Design review of the part built by this model. Coordinates are the model's own, in mm. Face numbers are marked on the shaded views. Round coordinates to 2 decimals unless told otherwise and drop trailing zeros. Loops run counter-clockwise (first coordinate to the right, second up) from the corner with the lowest first, then second, coordinate; pieces in that order, holes last. Notation, with made-up numbers: M -24,20.5 L -6,20.5 A26 ccw -6,38.5 Z; hole C 18,51 d3. An arc over 180 degrees is marked long. One line per item, written item: value. Start each with the question number.
Item 1: We need section C-C (z = 7.5). Write out the cut boundary in (x, y).
Item 2: We need section D-D (x = 14). Write out the cut boundary in (y, z).
Item 3: Clearance check with flat-ended pins moving along their axes: pin 1 (6.5 mm diameter, centred on x = -16.5, y = 15.5, fed in from +Z); pin 2 (1 mm diameter, centred on x = 18.5, z = 12.5, fed in from +Y); pin 3 (3.5 mm diameter, centred on x = 0.5, z = 1.5, fed in from -Y); pin 4 (1.5 mm diameter, centred on y = -15, z = 11.5, fed in from -X). State where each tip first meets the part, or that it passes through.
Item 4: For line 1 along X through (y, z) = (-20.5, 13); line 2 along X through (y, z) = (21.5, 7.75); line 3 along Y through (x, z) = (24, 14), list the stretches that pass through material, from the lowest coordinate up.
Item 5: We need section B-B (z = 13.75). Write out the cut boundary in (x, y), then the cut area to 3 significant figures.
Item 6: Mouldability with a two-part tool opening along X and no side actions: class the marked faces 1 and 2 as released by +X, released by -X, zero draft, split by the parting line, or undercut.
Item 7: We need section A-A (y = 0). Write out the cut boundary in (x, z), then the cut area to 3 significant figures.
from build123d import *

# Parameters (mm, degrees)
F0_W      = 55
F0_H      = 55
F1_DEPTH  = 3
F2_R      = 3.5
F3_DEPTH  = 3
F4_R      = 2.9
F5_DEPTH  = 3
F6_R      = 4.5
F7_DEPTH  = 12
F8_R      = 3.2
F9_DEPTH  = 12
F10_R     = 4
F11_W     = 15
F11_H     = 15
F12_DEPTH = 20
F14_DEPTH = 25
F15_R     = 8
F16_R     = 5


with BuildPart() as f1:
    # F0 (on Top) → F1 (new body)
    with BuildSketch(Plane.XY):
        Rectangle(F0_W, F0_H)
    extrude(amount=F1_DEPTH)

    # F2 (on face) → F3 (join)
    with BuildSketch(Plane.XY.offset(3)):
        with Locations((-15.9099025767, 15.9099025767)):
            Circle(F2_R)
        with Locations((15.9099025767, 15.9099025767)):
            Circle(F2_R)
        with Locations((-15.9099025767, -15.9099025767)):
            Circle(F2_R)
        with Locations((15.9099025767, -15.9099025767)):
            Circle(F2_R)
    extrude(amount=F3_DEPTH)

    # F4 (on face) → F5 (join)
    with BuildSketch(Plane.XY.offset(6)):
        with Locations((-15.9099025767, 15.9099025767)):
            Circle(F4_R)
        with Locations((15.9099025767, 15.9099025767)):
            Circle(F4_R)
        with Locations((-15.9099025767, -15.9099025767)):
            Circle(F4_R)
        with Locations((15.9099025767, -15.9099025767)):
            Circle(F4_R)
    extrude(amount=F5_DEPTH)

    # F6 (on face) → F7 (join)
    with BuildSketch(Plane.XY.offset(3)):
        with Locations((-22.627416998, 22.627416998)):
            Circle(F6_R)
        with Locations((22.627416998, 22.627416998)):
            Circle(F6_R)
        with Locations((22.627416998, -22.627416998)):
            Circle(F6_R)
        with Locations((-22.627416998, -22.627416998)):
            Circle(F6_R)
    extrude(amount=F7_DEPTH)

    # F8 (on face) → F9 (cut)
    with BuildSketch(Plane.XY.offset(15)):
        with Locations((-22.627416998, -22.627416998)):
            Circle(F8_R)
        with Locations((22.627416998, -22.627416998)):
            Circle(F8_R)
        with Locations((-22.627416998, 22.627416998)):
            Circle(F8_R)
        with Locations((22.627416998, 22.627416998)):
            Circle(F8_R)
    extrude(amount=-F9_DEPTH, mode=Mode.SUBTRACT)

    # F10
    f10_edges = [f1.edges().sort_by_distance(p)[0] for p in [
        (27.5, -27.5, 1.5),
        (-27.5, -27.5, 1.5),
        (-27.5, 27.5, 1.5),
        (27.5, 27.5, 1.5),
    ]]
    fillet(f10_edges, radius=F10_R)

    # F11 (on face) → F12 (cut, symmetric)
    with BuildSketch(Plane.XY.offset(3)):
        Polygon((-12.5, 4.5), (-27.5, 19.5), (-27.5, -19.5), (-12.5, -4.5), align=None)
        Polygon((19.5, 27.5), (-19.5, 27.5), (-4.5, 12.5), (4.5, 12.5), align=None)
        Polygon((27.5, -19.5), (27.5, 19.5), (12.5, 4.5), (12.5, -4.5), align=None)
        Polygon((-4.5, -12.5), (-19.5, -27.5), (19.5, -27.5), (4.5, -12.5), align=None)
        Rectangle(F11_W, F11_H)
    extrude(amount=F12_DEPTH, both=True, mode=Mode.SUBTRACT)

    # F13 (on face) → F14 (cut)
    with BuildSketch(Plane.XY.offset(3)):
        Polygon((-26.8456843913, 19.823363167), (-25.4314708289, 18.4091496047), (-22.6030437041, 21.2375767294), (-24.0172572665, 22.6517902918), align=None)
        Polygon((22.6030437041, 21.2375767294), (25.4314708289, 18.4091496047), (26.8456843913, 19.823363167), (24.0172572665, 22.6517902918), align=None)
        Polygon((-25.4314708289, -18.4091496047), (-26.8456843913, -19.823363167), (-24.0172572665, -22.6517902918), (-22.6030437041, -21.2375767294), align=None)
        Polygon((26.8456843913, -19.823363167), (25.4314708289, -18.4091496047), (22.6030437041, -21.2375767294), (24.0172572665, -22.6517902918), align=None)
    extrude(amount=F14_DEPTH, mode=Mode.SUBTRACT)

    # F15
    f15_edges = [f1.edges().sort_by_distance(p)[0] for p in [
        (19.5, -27.5, 1.5),
        (4.5, -12.5, 1.5),
        (-4.5, -12.5, 1.5),
        (-19.5, -27.5, 1.5),
        (-27.5, -19.5, 1.5),
        (-12.5, -4.5, 1.5),
        (-12.5, 4.5, 1.5),
        (-27.5, 19.5, 1.5),
        (-19.5, 27.5, 1.5),
        (-4.5, 12.5, 1.5),
        (4.5, 12.5, 1.5),
        (19.5, 27.5, 1.5),
        (12.5, -4.5, 1.5),
        (12.5, 4.5, 1.5),
        (27.5, 19.5, 1.5),
        (27.5, -19.5, 1.5),
    ]]
    fillet(f15_edges, radius=F15_R)

    # F16
    f16_edges = [f1.edges().sort_by_distance(p)[0] for p in [
        (-7.5, 7.5, 1.5),
        (7.5, 7.5, 1.5),
        (7.5, -7.5, 1.5),
        (-7.5, -7.5, 1.5),
    ]]
    fillet(f16_edges, radius=F16_R)


solid = f1.part
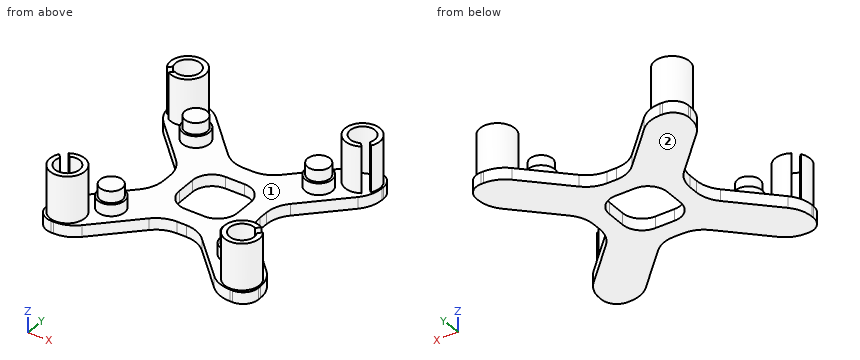
A:
1. outline: M -26.44,-20.23 A4.5 ccw long -25.02,-18.82 L -24.07,-19.77 A3.2 cw long -25.48,-21.19 Z; M -26.44,20.23 L -25.48,21.19 A3.2 cw long -24.07,19.77 L -25.02,18.82 A4.5 ccw long Z; C -15.91,-15.91 d5.8; C -15.91,15.91 d5.8; C 15.91,-15.91 d5.8; C 15.91,15.91 d5.8; M 24.07,-19.77 L 25.02,-18.82 A4.5 ccw long 26.44,-20.23 L 25.48,-21.19 A3.2 cw long Z; M 24.07,19.77 A3.2 cw long 25.48,21.19 L 26.44,20.23 A4.5 ccw long 25.02,18.82 Z
2. outline: M -22,0 L -5.85,0 L -5.85,3 L -12.98,3 L -12.98,6 L -13.73,6 L -13.73,9 L -18.09,9 L -18.09,6 L -18.84,6 L -18.84,3 L -22,3 Z; M 5.85,0 L 22,0 L 22,3 L 18.84,3 L 18.84,6 L 18.09,6 L 18.09,9 L 13.73,9 L 13.73,6 L 12.98,6 L 12.98,3 L 5.85,3 Z
3. pin 1: z = 9
3. pin 2: y = 25.29
3. pin 3: y = -12.57
3. pin 4: through
4. line 1: -26.59 to -26.17, -20.24 to -18.66, 18.66 to 20.24, 26.17 to 26.59
4. line 2: -26.98 to -25.62, -19.63 to -18.27, 18.27 to 19.63, 25.62 to 26.98
4. line 3: -26.91 to -25.52, -19.74 to -18.34, 18.34 to 19.74, 25.52 to 26.91
5. outline: M -26.44,-20.23 A4.5 ccw long -25.02,-18.82 L -24.07,-19.77 A3.2 cw long -25.48,-21.19 Z; M -26.44,20.23 L -25.48,21.19 A3.2 cw long -24.07,19.77 L -25.02,18.82 A4.5 ccw long Z; M 24.07,-19.77 L 25.02,-18.82 A4.5 ccw long 26.44,-20.23 L 25.48,-21.19 A3.2 cw long Z; M 24.07,19.77 A3.2 cw long 25.48,21.19 L 26.44,20.23 A4.5 ccw long 25.02,18.82 Z
5. area: 115 mm2
6. face 1: undercut
6. face 2: zero draft
7. outline: M -12.5,0 L -7.5,0 L -7.5,3 L -12.5,3 Z; M 7.5,0 L 12.5,0 L 12.5,3 L 7.5,3 Z
7. area: 30.0 mm2
